```python
from build123d import *

# Parameters (mm, degrees)
BOSS_EXTRUDE1_DEPTH = 3.175
SKETCH2_R           = 6.0325
BOSS_EXTRUDE2_DEPTH = 3.175
SKETCH3_R           = 1.5875
BOSS_EXTRUDE3_DEPTH = 3.175
FILLET1_R           = 2.54


with BuildPart() as part:
    # Sketch1 → Boss-Extrude1 (new body)
    with BuildSketch(Plane(origin=(0, 0, 0), x_dir=(1, 0, 0), z_dir=(0, 1, 0))):
        with BuildLine():
            Line((0, 0), (51.026830118, 0))
            Line((51.026830118, 0), (51.026830118, 25.4))
            Line((51.026830118, 25.4), (-0.321385748, 14.994382636))
            ThreePointArc((-0.321385748, 14.994382636), (-6.426220151, 7.362897615), (0, 0))
        make_face()
    extrude(amount=BOSS_EXTRUDE1_DEPTH)

    # Sketch2 → Boss-Extrude2 (add)
    with BuildSketch(Plane(origin=(0, 3.175, 0), x_dir=(1, 0, 0), z_dir=(0, 1, 0))):
        with Locations(Location((1.192030118, 7.526185235, 0), (0, 0, 270))):
            Circle(SKETCH2_R)
    extrude(amount=BOSS_EXTRUDE2_DEPTH)

    # Sketch3 → Boss-Extrude3 (add)
    with BuildSketch(Plane(origin=(0, 6.35, 0), x_dir=(1, 0, 0), z_dir=(0, 1, 0))):
        with Locations(Location((1.192030118, 7.526185235, 0), (0, 0, 270))):
            Circle(SKETCH3_R)
    extrude(amount=BOSS_EXTRUDE3_DEPTH)

    # Sketch5 → Revolve1 (revolve)
    with BuildSketch(Plane.XY.offset(-7.526185235)):
        with BuildLine():
            Line((1.250961313, 17.526), (1.250961313, 8.89))
            ThreePointArc((1.250961313, 8.89), (-3.067038687, 13.208), (1.250961313, 17.526))
        make_face()
    revolve(axis=Axis((1.250961313, 17.526, -7.526185235), (0, -1, 0)))

    # Fillet1
    fillet1_edges = [part.edges().sort_by_distance(p)[0] for p in [
        (51.026830118, 1.5875, 0),
        (51.026830118, 1.5875, -25.4),
    ]]
    fillet(fillet1_edges, radius=FILLET1_R)


solid = part.part
```
The listing builds one solid part. Answer for the finished solid, in the listing's coordinates (mm). A direction names the side the tool comes from. Coordinates: 2 decimals unless noted, no trailing zeros. Loops run counter-clockwise (first coordinate to the right, second up) from the corner with the lowest first, then second, coordinate; pieces in that order, holes last. Notation, with made-up numbers: M -31,39 L 3,39 A32 ccw 3,73 Z; hole C 78.5,85 d10. An arc over 180 degrees is marked long. Answer as a JSON object with one key per item and string values. Group by question number.
Item 1: Consider L1, parallel to Y at x = -2, z = -5.5; L2, parallel to Y at x = 39.5, z = -17 (3 decimals); L3, parallel to X at y = 6, z = -9. Determine where each line is inside the solid, lowest interval first.
Item 2: Section C-C (z = -8.5) is taken. Write down the section's boundary in (x, y) (3 decimals), and give its area (3 significant figures).
Item 3: Section B-B (y = 1.75) is taken. Write down the section's boundary in (x, z), and give its area (3 significant figures).
Item 4: Each of these flat-tipped pins is pushed along its axis until it touches: P1, Ø3, axis at x = 26, y = 3.5, coming from the -Z side; P2, Ø1, axis at x = 13, z = -18.5, coming from the +Y side; P3, Ø5, axis at y = 6, z = -4, coming from the -X side; P4, Ø7.5, axis at x = 25, z = -14, coming from the +Y side (3 decimals). Where does it stop, or does it pass through?
Item 5: Determine the mould class of faces 4 (the face through (0, 6.35, -6)), 5 (the face through (28, 3.175, -10)), 6 (the face through (22, 0, -10)), 7 (the face through (51.027, 2, -12)) for opening direction Y: +Y half, -Y half, draft (parallel to the pull), parting line (faces both ways), or undercut.
Item 6: Which of the six approach directions +Z, -Z, +X, -X, +Y, -Y give full straight-line access (tool end or side, diameter ignored) to faces 1 (the face through (-2.48, 4.74, -12.31)), 2 (the face through (1.669, 7.763, -6.012)), 3 (the face through (50.26, 1.61, -0.72))?
Item 7: Section A-A (z = -5) is taken. Write down the section's boundary in (x, y) (3 decimals).
Item 8: Section D-D (x = 9.5) is taken. Write down the section's boundary in (y, z) (3 decimals), and give its area (3 significant figures).
Solved:
{
 "1": {"L1": "y = 0 to 6.35, 11.22 to 15.2", "L2": "y = 0 to 3.175", "L3": "x = -4.66 to 7.04"},
 "2": {"outline": "M -6.365,0 L 51.027,0 L 51.027,3.175 L 7.145,3.175 L 7.145,6.35 L 2.446,6.35 L 2.446,9.174 A4.207 ccw long -0.062,9.211 L -0.062,6.35 L -4.761,6.35 L -4.761,3.175 L -6.365,3.175 Z", "area": "282 mm2"},
 "3": {"outline": "M -0.32,-14.99 L 47.98,-24.78 A2.54 ccw 51.03,-22.29 L 51.03,-2.54 A2.54 ccw 48.49,0 L 0,0 A7.62 ccw Z", "area": "1,100 mm2"},
 "4": {"P1": "stops at z = -20.63", "P2": "passes through", "P3": "stops at x = -4.75", "P4": "stops at y = 3.175"},
 "5": {"face 4": "undercut", "face 5": "+Y half", "face 6": "-Y half", "face 7": "draft"},
 "6": {"face 1": "+Y", "face 2": "none", "face 3": "+Z, +X, +Y, -Y"},
 "7": {"outline": "M -5.997,0 L 51.027,0 L 51.027,3.175 L 6.67,3.175 L 6.67,6.35 L -4.286,6.35 L -4.286,3.175 L -5.997,3.175 Z; C 1.251,13.208 d7.004"},
 "8": {"outline": "M 0,-16.985 L 3.175,-16.985 L 3.175,0 L 0,0 Z", "area": "53.9 mm2"}
}
